```python
from build123d import *

# Parameters (mm, degrees)
SKETCH_1_R      = 0.4
EXTRUDE_1_DEPTH = 10
SKETCH_2_W      = 70
SKETCH_2_H      = 0.8
EXTRUDE_2_DEPTH = 0.8
FILLET_1_R      = 0.4
SKETCH_3_R      = 0.4
EXTRUDE_3_DEPTH = 5
SKETCH_4_R      = 0.4
EXTRUDE_4_DEPTH = 5
CHAMFER_1_SIZE  = 0.4


with BuildPart() as part:
    # 草图1 → 凸台-拉伸1 (new body)
    with BuildSketch(Plane(origin=(0, 0, 0), x_dir=(1, 0, 0), z_dir=(0, 1, 0))):
        with Locations(Location((0, 0, 0), (0, 0, 270))):
            Circle(SKETCH_1_R)
    extrude(amount=EXTRUDE_1_DEPTH)

    # 草图2 → 凸台-拉伸2 (add)
    with BuildSketch(Plane(origin=(0, 10, 0), x_dir=(1, 0, 0), z_dir=(0, 1, 0))):
        Rectangle(SKETCH_2_W, SKETCH_2_H)
    extrude(amount=EXTRUDE_2_DEPTH)

    # 圆角1
    fillet_1_edges = [part.edges().sort_by_distance(p)[0] for p in [
        (35, 10, 0),
        (35, 10.8, 0),
        (-35, 10, 0),
        (-35, 10.8, 0),
    ]]
    fillet(fillet_1_edges, radius=FILLET_1_R - 0.0001)  # a hair under: the kernel refuses the full size

    # 草图3 → 凸台-拉伸3 (add)
    with BuildSketch(Plane.XY.offset(0.4)):
        with Locations((34.6, 10.4)):
            Circle(SKETCH_3_R)
    extrude(amount=EXTRUDE_3_DEPTH)

    # 草图4 → 凸台-拉伸4 (add)
    with BuildSketch(Plane(origin=(0, 0, -0.4), x_dir=(-1, 0, 0), z_dir=(0, 0, -1))):
        with Locations((34.6, 10.4)):
            Circle(SKETCH_4_R)
    extrude(amount=EXTRUDE_4_DEPTH)

    # 倒角1
    chamfer_1_edges = [part.edges().sort_by_distance(p)[0] for p in [
        (34.2, 10.4, 5.4),
        (-34.2, 10.4, -5.4),
    ]]
    chamfer(chamfer_1_edges, length=CHAMFER_1_SIZE - 0.0001)  # a hair under: the kernel refuses the full size


solid = part.part
```
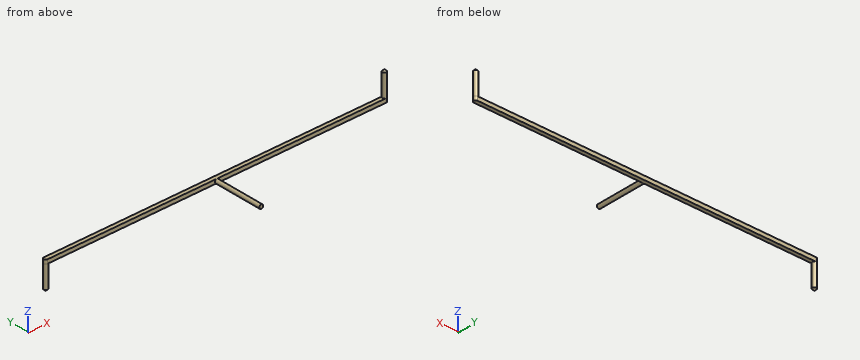
Model file for the job. Use its own axes, mm. Coordinates: 2 decimals unless noted, no trailing zeros. Order: outer loops, then holes, each group sorted by start corner. A loop starts at its lowest first (then second) coordinate and runs counter-clockwise, first axis right, second up. Notation, with made-up numbers: (8.25, 18.5) - (62.25, 18.5) arc R28 ccw to (62.25, 54.5) - close; hole circle Ø6 at (-34, 53). An arc over 180 degrees is marked (long way). Return JSON: item names as keys, results as strings. Group by question number.
1) Flat gauge pins, fed straight in: P1, Ø6, axis at y = 4, z = 2, coming from the -X side; P2, Ø0.9, axis at x = 1, y = 10.5, coming from the -Z side; P3, Ø4, axis at x = -1.5, y = 8.5, coming from the +Z side. Where does each tip first touch, or does it go through?
2) Saw through at A-A, the plane x = -3. Write the cut outline in (y, z), plus the area to 3 significant figures.
3) Saw through at B-B, the plane y = 5.5. Write the cut outline in (x, z).
4) Saw through at C-C, the plane z = 2.5. Write the cut outline in (x, y), plus the area to 3 significant figures.
Values found:
{
 "1": {"P1": "stops at x = -0.4", "P2": "stops at z = -0.4", "P3": "stops at z = 0.4"},
 "2": {"outline": "(10, -0.4) - (10.8, -0.4) - (10.8, 0.4) - (10, 0.4) - close", "area": "0.640 mm²"},
 "3": {"outline": "circle Ø0.8 at (0, 0)"},
 "4": {"outline": "circle Ø0.8 at (34.6, 10.4)", "area": "0.503 mm²"}
}
